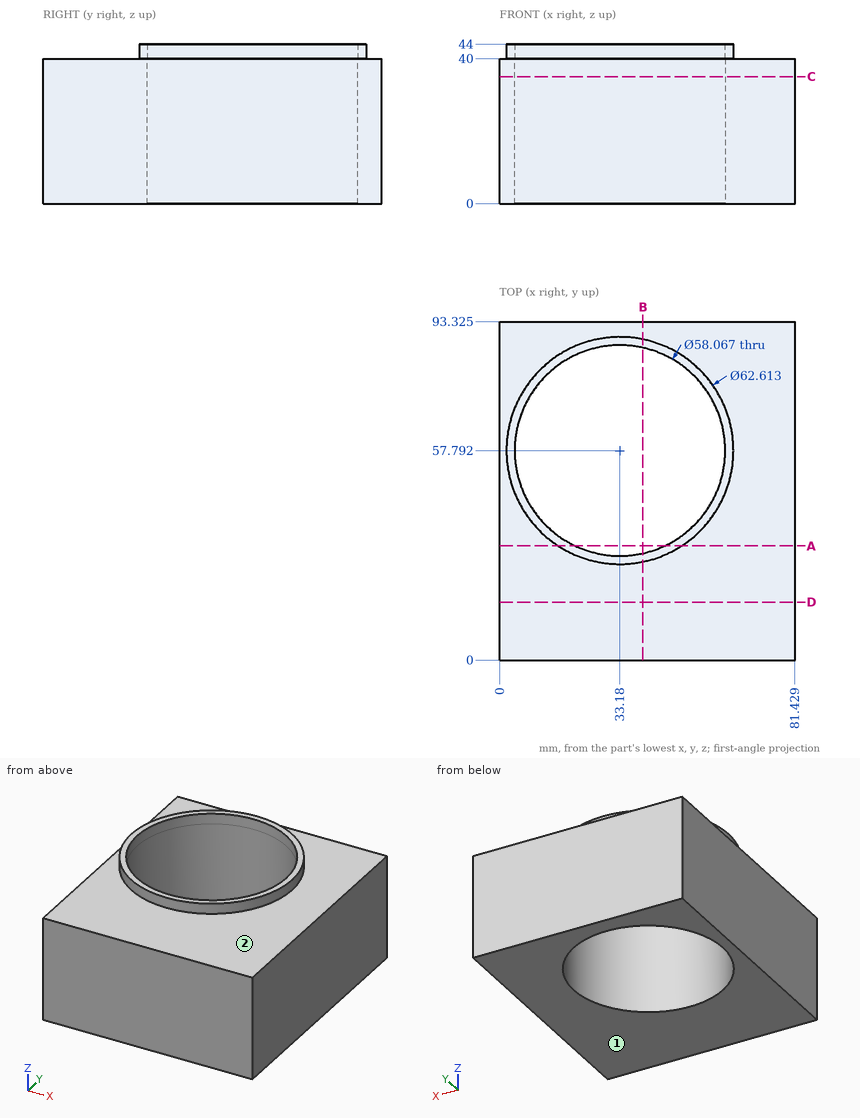
Drawing for the job (mm, zero at the part's lowest x, y, z). A direction names the side the tool comes from. Coordinates: 2 decimals unless noted, no trailing zeros. Loops run counter-clockwise (first coordinate to the right, second up) from the corner with the lowest first, then second, coordinate; pieces in that order, holes last. Notation, with made-up numbers: (41.5, 15) - (54.5, 15) arc R28 cw to (54.5, 41) - close; hole circle Ø8 at (9.5, -25.75). An arc over 180 degrees is marked (long way). Return JSON: item names as keys, results as strings.
1. Band-saw the part on C-C (z = 35). Give the cut face in (x, y) (1 decimal).
Result:
{"outline": "(0, 0) - (81.4, 0) - (81.4, 93.3) - (0, 93.3) - close; hole circle Ø58.1 at (33.2, 57.8)"}
2. Band-saw the part on D-D (y = 16). Give the cut face in (x, z).
Result:
{"outline": "(0, 0) - (81.43, 0) - (81.43, 40) - (0, 40) - close"}
3. Band-saw the part on B-B (x = 39.5). Give the cut face in (y, z) (1 decimal), and give its area (3 significant figures).
Result:
{"outline": "(0, 0) - (29.5, 0) - (29.5, 44) - (27.1, 44) - (27.1, 40) - (0, 40) - close; (86.1, 0) - (93.3, 0) - (93.3, 40) - (88.5, 40) - (88.5, 44) - (86.1, 44) - close", "area": "1,480 mm2"}
4. 3-axis set-ups, long thin cutter, end or side, ignore diameter. For the marked faces 1 and 2: which of +Z, -Z, +X, -X, +Y, -Y reach the whole face in a straight line?
Result:
{"face 1": "-Z, +X, -X, +Y, -Y", "face 2": "+Z"}
5. Band-saw the part on A-A (y = 31.5). Give the cut face in (x, z) (1 decimal).
Result:
{"outline": "(0, 0) - (20.9, 0) - (20.9, 44) - (16.2, 44) - (16.2, 40) - (0, 40) - close; (45.5, 0) - (81.4, 0) - (81.4, 40) - (50.2, 40) - (50.2, 44) - (45.5, 44) - close"}
6. Probe L1, parallel to Y at x = 32.5, z = 33.5 (1 decimal); L2, parallel to Y at x = 49, z = 24 (1 decimal); L3, parallel to Z at x = 57.5, y = 36. List the from-to ranges inside material, lowest first. Write a range as from..to.
Result:
{"L1": "y = 0..28.8, 86.8..93.3", "L2": "y = 0..33.4, 82.1..93.3", "L3": "z = 0..40"}
7. Drop flat-ended pins along their axis: pin 1 (4 mm diameter, centred on x = 60, y = 64, fed in from -Z); pin 2 (6 mm diameter, centred on x = 23, y = 21.5, fed in from +Z); pin 3 (6 mm diameter, centred on x = 56.5, y = 50.5, fed in from +Z). Give the stop position or say it passes through.
Result:
{"pin 1": "stops at z = 0", "pin 2": "stops at z = 40", "pin 3": "passes through"}
